Here's how the part is built. I have some questions about the finished solid (model axes, mm). Face numbers are marked on the shaded views. Round coordinates to 2 decimals unless told otherwise and drop trailing zeros. Loops run counter-clockwise (first coordinate to the right, second up) from the corner with the lowest first, then second, coordinate; pieces in that order, holes last. Notation, with made-up numbers: M 29.25,75 L 41.25,75 A17 ccw 41.25,99 Z; hole C 62.5,-22.5 d4. An arc over 180 degrees is marked long. Answer as a JSON object with one key per item and string values.
from build123d import *

# Parameters (mm, degrees)
SKETCH2_W                                       = 65.110000082
SKETCH2_H                                       = 42
BOSS_EXTRUDE1_DEPTH                             = 9.525
CSK_FOR_10_FLAT_HEAD_MACHINE_SCREW1_D           = 5.1054
CSK_FOR_10_FLAT_HEAD_MACHINE_SCREW1_CSINK_D     = 9.779
CSK_FOR_10_FLAT_HEAD_MACHINE_SCREW1_CSINK_ANGLE = 82
SKETCH15_W                                      = 3.175
SKETCH15_H                                      = 6.35
CUT_EXTRUDE1_DEPTH                              = 79.064317942
ADVANCEDHOLE2_OUTLINE_R                         = 2.0193
ADVANCEDHOLE2_DEPTH                             = 9.525


# Read off the part's stored shape, not the designer's step: AdvancedHole2
with BuildPart() as part:
    # Sketch2 → Boss-Extrude1 (new body)
    with BuildSketch(Plane(origin=(0, 0, 0), x_dir=(1, 0, 0), z_dir=(0, 1, 0))):
        with Locations((-32.555000041, 21)):
            Rectangle(SKETCH2_W, SKETCH2_H)
    extrude(amount=BOSS_EXTRUDE1_DEPTH)

    # CSK for #10 Flat Head Machine Screw1 (through all)
    with Locations(Plane(origin=(0, 9.525, 0), x_dir=(1, 0, 0), z_dir=(0, 1, 0))):
        with Locations((-54.830000082, 33.7), (-54.830000082, 8.3), (-10.3799894, 8.3), (-10.3799894, 33.7)):
            CounterSinkHole(CSK_FOR_10_FLAT_HEAD_MACHINE_SCREW1_D / 2, CSK_FOR_10_FLAT_HEAD_MACHINE_SCREW1_CSINK_D / 2, counter_sink_angle=CSK_FOR_10_FLAT_HEAD_MACHINE_SCREW1_CSINK_ANGLE)

    # Sketch15 → Cut-Extrude1 (cut, through all)
    with BuildSketch(Plane(origin=(0, 9.525, 0), x_dir=(1, 0, 0), z_dir=(0, 1, 0))):
        with Locations((-63.522500082, 21)):
            Rectangle(SKETCH15_W, SKETCH15_H)
    extrude(amount=-CUT_EXTRUDE1_DEPTH, mode=Mode.SUBTRACT)

    # AdvancedHole2 outline → AdvancedHole2 (cut)
    with BuildSketch(Plane(origin=(0, 0, 0), x_dir=(1, 0, 0), z_dir=(0, 1, 0))):
        with Locations((-33.600000082, 8.3)):
            Circle(ADVANCEDHOLE2_OUTLINE_R)
        with Locations((-33.600000082, 33.7)):
            Circle(ADVANCEDHOLE2_OUTLINE_R)
    extrude(amount=ADVANCEDHOLE2_DEPTH, mode=Mode.SUBTRACT)


solid = part.part
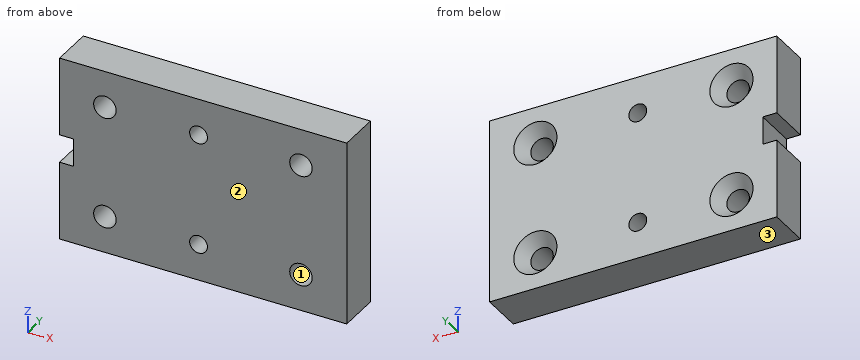
Item 1: I want a section at C-C, the plane y = 2.75. Please give me the cut outline in (x, z) (3 decimals).
Resolved:
{"outline": "M -65.11,-42 L 0,-42 L 0,0 L -65.11,0 L -65.11,-17.825 L -61.935,-17.825 L -61.935,-24.175 L -65.11,-24.175 Z; hole C -54.83,-33.7 d5.105; hole C -54.83,-8.3 d5.105; hole C -33.6,-33.7 d4.039; hole C -33.6,-8.3 d4.039; hole C -10.38,-33.7 d5.105; hole C -10.38,-8.3 d5.105"}
Item 2: I want a section at B-B, the plane z = -33.7. Please give me the cut outline in (x, y) (1 decimal), then the cut area to 3 significant figures.
Resolved:
{"outline": "M -65.1,0 L -57.4,0 L -57.4,6.8 L -59.7,9.5 L -65.1,9.5 Z; M -52.3,0 L -35.6,0 L -35.6,9.5 L -49.9,9.5 L -52.3,6.8 Z; M -31.6,0 L -12.9,0 L -12.9,6.8 L -15.3,9.5 L -31.6,9.5 Z; M -7.8,0 L 0,0 L 0,9.5 L -5.5,9.5 L -7.8,6.8 Z", "area": "472 mm²"}
Item 3: I'm going to push flat-ended pins straight in: pin 1 Ø3 at (y, z) = (4.5, -20.5) entering from -X (3 decimals); pin 2 Ø3 at (x, z) = (-54.83, -33.7) entering from +Y; pin 3 Ø6 at (x, z) = (-10.38, -8.3) entering from +Y. Where does each tip first touch, or does it pass through?
Resolved:
{"pin 1": "x = -61.935", "pin 2": "through", "pin 3": "y = 7.35"}
Item 4: I want a section at D-D, the plane y = 8.25. Please give me the cut outline in (x, z) (3 decimals).
Resolved:
{"outline": "M -65.11,-42 L 0,-42 L 0,0 L -65.11,0 L -65.11,-17.825 L -61.935,-17.825 L -61.935,-24.175 L -65.11,-24.175 Z; hole C -54.83,-33.7 d7.562; hole C -54.83,-8.3 d7.562; hole C -33.6,-33.7 d4.039; hole C -33.6,-8.3 d4.039; hole C -10.38,-33.7 d7.562; hole C -10.38,-8.3 d7.562"}
Item 5: If we mould it in two halves opening along Z, with no side actions, what happens to the marked faces 1, 2 and 3? For each: pulls with the +Z half, pulls with the -Z half, needs draft (parallel to the pull), parting line crosses it, or undercut.
Resolved:
{"face 1": "undercut", "face 2": "needs draft", "face 3": "pulls with the -Z half"}
Item 6: I want a section at A-A, the plane x = -33.6. Please give me the cut outline in (y, z) (3 decimals).
Resolved:
{"outline": "M 0,-42 L 9.525,-42 L 9.525,-35.719 L 0,-35.719 Z; M 0,-31.681 L 9.525,-31.681 L 9.525,-10.319 L 0,-10.319 Z; M 0,-6.281 L 9.525,-6.281 L 9.525,0 L 0,0 Z"}
Item 7: Please list where these lines run through material, in increasing order: probe 1 along X at (y, z) = (4.25, -33.7); probe 2 along Z at (x, y) = (-54.83, 3.75); probe 3 along X at (y, z) = (5.75, -10). Write a range as from..to.
Resolved:
{"probe 1": "-65.11..-57.38, -52.28..-35.62, -31.58..-12.93, -7.83..0", "probe 2": "-42..-36.25, -31.15..-10.85, -5.75..0", "probe 3": "-65.11..-56.73, -52.93..-34.69, -32.51..-12.28, -8.48..0"}
